Build history of the part. All positions in model axes, mm. A direction names the side the tool comes from. Coordinates: 2 decimals unless noted, no trailing zeros. Loops run counter-clockwise (first coordinate to the right, second up) from the corner with the lowest first, then second, coordinate; pieces in that order, holes last.
(1) Slice it at B-B (x = -37.5). Give the cut face in (y, z), and give its area (3 significant figures).
(2) Slice it at D-D (y = 0). Give the cut face in (x, z).
(3) Tool access for faces 1 (the face through (-11.53, -12.08, 4.94)), 2 (the face through (-40.553, -10.726, 5.076)), 3 (the face through (-4, -20.8, 1.4)), 4 (the face through (-40, 15, 5)): list every direction of +Z, -Z, +X, -X, +Y, -Y with a clear straight run to the whole face (end or side of a thin tool).
(4) Flat gauge pins, fed straight in: P1, Ø4, axis at x = -31, z = 3.5, coming from the -Y side; P2, Ø5.5, axis at y = -22, z = 5, coming from the -X side; P3, Ø4, axis at y = 19, z = 8.5, coming from the -X side. Where does each tip first touch, or does it go through?
(5) Slice it at C-C (z = 5). Give the number of separate pieces and of enclosed holes in the cut face, and give its area (3 significant figures).
(6) Two-plate mould, pull along X, no slides. Class faces 5 (the face through (-1.397, 20.185, 3.843)), 6 (the face through (-38.1, -12.3, 4.9)), 7 (the face through (-27, 5, 5)), 8 (the face through (-42.1, 0, 5)): pulls with the +X half, pulls with the -X half, needs draft (parallel to the pull), parting line crosses it, or undercut.
(7) Slice it at A-A (y = 22). Give the cut face in (x, z).
(8) Wall check: L1, parallel to Z at x = -2.15, y = 22; L2, parallel to Y at x = -1.5, z = 5; L3, parallel to Y at x = -24, z = 8.75. Give the ranges that are in metal, low to high.
from build123d import *

# Parameters (mm, degrees)
SKETCH1_R                                         = 16.7
SKETCH1_R_2                                       = 12.7
BOSS_EXTRUDE1_DEPTH                               = 10
SKETCH2_W                                         = 22.16607393
SKETCH2_H                                         = 10
SKETCH2_W_2                                       = 4
SKETCH2_H_2                                       = 30
BOSS_EXTRUDE2_DEPTH                               = 10
SKETCH4_W                                         = 8
SKETCH4_H                                         = 11.78611706
BOSS_EXTRUDE3_DEPTH                               = 10
FILLET3_R                                         = 1
CSK_FOR_6_FLAT_HEAD_MACHINE_SCREW_100_D           = 4.3053
CSK_FOR_6_FLAT_HEAD_MACHINE_SCREW_100_CSINK_D     = 7.0866
CSK_FOR_6_FLAT_HEAD_MACHINE_SCREW_100_CSINK_ANGLE = 100
INTERSECT3_OUTLINE_R                              = 2.15265
INTERSECT3_DEPTH                                  = 16.7


# Read off the part's stored shape, not the designer's step: CSK for #4 Flat Head Machine Screw (100)1, Intersect3
with BuildPart() as part:
    # Sketch1 → Boss-Extrude1 (new body)
    with BuildSketch(Plane.XY):
        Circle(SKETCH1_R)
        Circle(SKETCH1_R_2, mode=Mode.SUBTRACT)
    extrude(amount=BOSS_EXTRUDE1_DEPTH)

    # Sketch2 → Boss-Extrude2 (add)
    with BuildSketch(Plane(origin=(0, 0, 0), x_dir=(-1, 0, 0), z_dir=(0, 0, -1))):
        with Locations((27.016963035, 0)):
            Rectangle(SKETCH2_W, SKETCH2_H)
        with Locations((40.1, 0)):
            Rectangle(SKETCH2_W_2, SKETCH2_H_2)
    extrude(amount=-BOSS_EXTRUDE2_DEPTH)

    # Sketch4 → Boss-Extrude3 (add)
    with BuildSketch(Plane(origin=(0, 0, 0), x_dir=(-1, 0, 0), z_dir=(0, 0, -1))):
        with Locations((0, 22.10694147)):
            Rectangle(SKETCH4_W, SKETCH4_H)
    boss_extrude3 = extrude(amount=-BOSS_EXTRUDE3_DEPTH)

    # Mirror1: Boss-Extrude3 across plane
    add(boss_extrude3.mirror(Plane.ZX))

    # Fillet3
    fillet3_edges = [part.edges().sort_by_distance(p)[0] for p in [
        (-11.435827246, -12.170121413, 10),
        (-11.435827246, -12.170121413, 0),
        (-38.1, 10, 10),
        (-40.1, -15, 10),
        (-27.016963035, -5, 10),
        (-38.1, -10, 0),
        (-40.1, 15, 0),
        (-38.1, 10, 0),
        (-27.016963035, 5, 0),
        (-38.1, -10, 10),
        (-40.1, -15, 0),
        (-40.1, 15, 10),
        (-15.93392607, -5, 5),
        (-27.016963035, -5, 0),
        (-27.016963035, 5, 10),
        (-15.93392607, 5, 5),
        (-11.435827246, 12.170121413, 0),
        (-11.435827246, 12.170121413, 10),
        (-4, 22.10694147, 0),
        (0, 28, 0),
        (4, 22.10694147, 0),
        (0, 28, 10),
        (4, 28, 5),
        (4, 22.10694147, 10),
        (4, 16.21388294, 5),
        (-4, 16.21388294, 5),
        (-4, 22.10694147, 10),
        (-4, 28, 5),
        (16.7, 0, 0),
        (16.7, 0, 10),
        (-4, -16.21388294, 5),
        (-4, -22.10694147, 0),
        (-4, -28, 5),
        (0, -28, 0),
        (4, -28, 5),
        (4, -22.10694147, 0),
        (4, -16.21388294, 5),
        (-4, -22.10694147, 10),
        (0, -28, 10),
        (4, -22.10694147, 10),
    ]]
    fillet(fillet3_edges, radius=FILLET3_R)

    # CSK for _4 Flat Head Machine Screw _ 2 → CSK for #4 Flat Head Machine Screw (100)1 (revolve, cut)
    with BuildSketch(Plane(origin=(0, -9, 5), x_dir=(0, 1, 0), z_dir=(0, 0, -1))):
        Polygon((0, -42.1), (1.7272, -42.1), (1.7272, -39.048434313), (2.8575, -38.1), (0, -38.1), align=None)
    csk_for_4_flat_head_machine_screw_100 = revolve(axis=Axis((0, -9, 5), (1, 0, 0)), mode=Mode.SUBTRACT)

    # Mirror2: CSK for #4 Flat Head Machine Screw (100)1 across plane
    add(csk_for_4_flat_head_machine_screw_100.mirror(Plane.ZX), mode=Mode.SUBTRACT)

    # CSK for #6 Flat Head Machine Screw (100)5 (through all)
    with Locations(Plane.ZY.offset(4)):
        with Locations((5, -22)):
            csk_for_6_flat_head_machine_screw_100 = CounterSinkHole(CSK_FOR_6_FLAT_HEAD_MACHINE_SCREW_100_D / 2, CSK_FOR_6_FLAT_HEAD_MACHINE_SCREW_100_CSINK_D / 2, counter_sink_angle=CSK_FOR_6_FLAT_HEAD_MACHINE_SCREW_100_CSINK_ANGLE)

    # Mirror5: CSK for #6 Flat Head Machine Screw (100)5 across plane
    add(csk_for_6_flat_head_machine_screw_100.mirror(Plane.ZX), mode=Mode.SUBTRACT)

    # Intersect3 outline → Intersect3 (cut)
    with BuildSketch(Plane.YZ):
        with BuildLine():
            ThreePointArc((28, 9), (27.707106781, 9.707106781), (27, 10))
            Line((27, 10), (-27, 10))
            ThreePointArc((-27, 10), (-27.707106781, 9.707106781), (-28, 9))
            Line((-28, 9), (-28, 1))
            ThreePointArc((-28, 1), (-27.707106781, 0.292893219), (-27, 0))
            Line((-27, 0), (27, 0))
            ThreePointArc((27, 0), (27.707106781, 0.292893219), (28, 1))
            Line((28, 1), (28, 9))
        make_face()
        with Locations((-22, 5)):
            Circle(INTERSECT3_OUTLINE_R, mode=Mode.SUBTRACT)
        with Locations((22, 5)):
            Circle(INTERSECT3_OUTLINE_R, mode=Mode.SUBTRACT)
    extrude(amount=INTERSECT3_DEPTH, mode=Mode.SUBTRACT)


solid = part.part
Response values:
1. outline: (-5, 1) arc R1 ccw to (-4, 0) - (4, 0) arc R1 ccw to (5, 1) - (5, 9) arc R1 ccw to (4, 10) - (-4, 10) arc R1 ccw to (-5, 9) - close
1. area: 99.1 mm2
2. outline: (-42.1, 0) - (-12.7, 0) - (-12.7, 10) - (-42.1, 10) - close
3. face 1: +Z, -Z, -Y
3. face 2: -X
3. face 3: +Z, -Z, -X, -Y
3. face 4: +Z, -Z, -X, +Y
4. P1: stops at y = -5
4. P2: stops at x = -3.33
4. P3: stops at x = -4
5. separate pieces: 5
5. enclosed holes: 0
5. area: 545 mm2
6. face 5: needs draft
6. face 6: undercut
6. face 7: undercut
6. face 8: pulls with the -X half
7. outline: (-4, 1) arc R1 ccw to (-3, 0) - (0, 0) - (0, 2.85) - (-2.83, 2.85) - (-4, 1.46) - close; (-4, 8.54) - (-2.83, 7.15) - (0, 7.15) - (0, 10) - (-3, 10) arc R1 ccw to (-4, 9) - close
8. L1: z = 0 to 2.85, 7.15 to 10
8. L2: y = -28 to -24.15, -19.85 to -12.61, 12.61 to 19.85, 24.15 to 28
8. L3: y = -5 to 5
